Could you check a few things on this model? Use its own coordinates, in mm. A direction names the side the tool comes from. Coordinates: 2 decimals unless noted, no trailing zeros. Loops run counter-clockwise (first coordinate to the right, second up) from the corner with the lowest first, then second, coordinate; pieces in that order, holes last. Notation, with made-up numbers: (-34.75, 34.25) -> (-1.75, 34.25) arc R16 cw to (-1.75, 42.25) -> close; hole circle Ø7 at (76.25, 1.25). An arc over 180 degrees is marked (long way). One line per question, with ' | ' between items.
from build123d import *

# Parameters (mm, degrees)
SKETCH1_W            = 224.79
SKETCH1_H            = 146.05
BOSS_EXTRUDE1_DEPTH  = 1.98374
SKETCH2_W            = 20.32
SKETCH2_H            = 20.32
SKETCH2_H_2          = 1.27
CORNER_CUT_DEPTH     = 135.049326274
SKETCH3_R            = 2.159
PS_MOUNT_HOLES_DEPTH = 135.049326274
PS_CUTOUT_DEPTH      = 135.049326274
FILLET11_R           = 6.35
SKETCH5_R            = 2.8956
FRAME_MOUNTS_DEPTH   = 135.049326274
SKETCH8_W            = 204.47
SKETCH8_H            = 19.05
BOSS_EXTRUDE2_DEPTH  = 1.98374


with BuildPart() as part:
    # Sketch1 → Boss-Extrude1 (new body)
    with BuildSketch(Plane.XY):
        Rectangle(SKETCH1_W, SKETCH1_H)
    extrude(amount=BOSS_EXTRUDE1_DEPTH)

    # Sketch2 → Corner Cut (cut, through all)
    with BuildSketch(Plane.XY.offset(1.98374)):
        with Locations((-102.235, 62.865)):
            Rectangle(SKETCH2_W, SKETCH2_H)
        with Locations((-102.235, -72.39)):
            Rectangle(SKETCH2_W, SKETCH2_H_2)
    extrude(amount=-CORNER_CUT_DEPTH, mode=Mode.SUBTRACT)

    # Sketch3 → PS Mount Holes (cut, through all)
    with BuildSketch(Plane.XY.offset(1.98374)):
        with Locations((-86.075, 46.705)):
            Circle(SKETCH3_R)
        with Locations((-62.0776, -27.295)):
            Circle(SKETCH3_R)
        with Locations((39.925000098, -17.295)):
            Circle(SKETCH3_R)
        with Locations((39.925000098, 46.705)):
            Circle(SKETCH3_R)
    extrude(amount=-PS_MOUNT_HOLES_DEPTH, mode=Mode.SUBTRACT)

    # Sketch4 → PS Cutout (cut, through all)
    with BuildSketch(Plane.XY.offset(1.98374)):
        Polygon((-77.185, 55.595), (31.035000098, 55.595), (31.035000098, 37.815), (48.815000098, 37.815), (48.815000098, -8.405), (31.035000098, -8.405), (31.035000098, -36.185), (-53.1876, -36.185), (-53.1876, -18.405), (-94.965, -18.405), (-94.965, 37.815), (-77.185, 37.815), align=None)
    extrude(amount=-PS_CUTOUT_DEPTH, mode=Mode.SUBTRACT)

    # Fillet11
    fillet11_edges = [part.edges().sort_by_distance(p)[0] for p in [
        (-77.185, 37.815, 0.99187),
        (-77.185, 55.595, 0.99187),
        (31.035000098, 55.595, 0.99187),
        (31.035000098, 37.815, 0.99187),
        (48.815000098, 37.815, 0.99187),
        (48.815000098, -8.405, 0.99187),
        (31.035000098, -8.405, 0.99187),
        (31.035000098, -36.185, 0.99187),
        (-53.1876, -36.185, 0.99187),
        (-53.1876, -18.405, 0.99187),
        (-94.965, -18.405, 0.99187),
        (-94.965, 37.815, 0.99187),
    ]]
    fillet(fillet11_edges, radius=FILLET11_R)

    # Sketch5 → Frame-Mounts (cut, through all)
    with BuildSketch(Plane.XY.offset(1.98374)):
        with Locations((-62.865, 64.77)):
            Circle(SKETCH5_R)
        with Locations((76.835, 64.77)):
            Circle(SKETCH5_R)
        with Locations((-104.14, -36.83)):
            Circle(SKETCH5_R)
    extrude(amount=-FRAME_MOUNTS_DEPTH, mode=Mode.SUBTRACT)

    # Sketch8 → Boss-Extrude2 (add)
    with BuildSketch(Plane.XZ.offset(73.025)):
        with Locations((10.16, -7.54126)):
            Rectangle(SKETCH8_W, SKETCH8_H)
    extrude(amount=BOSS_EXTRUDE2_DEPTH)


solid = part.part
1) On a 3-axis mill with a long thin cutter (end or side, diameter ignored), from which of +Z, -Z, +X, -X, +Y, -Y can I reach the whole of each face in a straight line? I mean faces 1 (the face through (112.395, -1, 1)), 2 (the face through (32.94, 39.63, 0.98)), 3 (the face through (9, -73.025, -8)). Say none if no direction works.
Data:
face 1: +Z, -Z, +X, +Y, -Y | face 2: +Z, -Z | face 3: -Z, +X, -X, +Y
2) If we section it at B-B on y = 64.77: Please give me the cut outline in (x, z) (3 decimals).
Data:
outline: (-92.075, 0) -> (-65.761, 0) -> (-65.761, 1.984) -> (-92.075, 1.984) -> close; (-59.969, 0) -> (73.939, 0) -> (73.939, 1.984) -> (-59.969, 1.984) -> close; (79.731, 0) -> (112.395, 0) -> (112.395, 1.984) -> (79.731, 1.984) -> close
3) If we section it at D-D on x = -26.5: Please give me the cut outline in (y, z) (3 decimals).
Data:
outline: (-75.009, -17.066) -> (-73.025, -17.066) -> (-73.025, 0) -> (-36.185, 0) -> (-36.185, 1.984) -> (-75.009, 1.984) -> close; (55.595, 0) -> (73.025, 0) -> (73.025, 1.984) -> (55.595, 1.984) -> close
4) If we section it at C-C on x = 90.5: Please give me the cut outline in (y, z) (3 decimals).
Data:
outline: (-75.009, -17.066) -> (-73.025, -17.066) -> (-73.025, 0) -> (73.025, 0) -> (73.025, 1.984) -> (-75.009, 1.984) -> close
5) We'd pull the mould along Y, two halves only. Please class faces 4 (the face through (48, -16, 1.984)), 5 (the face through (9, -75.009, -7)), 6 (the face through (47, 35.91, 0.98)): pulls with the +Y half, pulls with the -Y half, needs draft (parallel to the pull), parting line crosses it, or undercut.
Data:
face 4: needs draft | face 5: pulls with the -Y half | face 6: undercut
6) I'm going to push flat-ended pins straight in: pin 1 Ø9.5 at (x, y) = (76.835, 64.77) entering from -Z; pin 2 Ø1.6 at (y, z) = (-74, -7.5) entering from -X (3 decimals); pin 3 Ø5 at (x, z) = (-87, -6.5) entering from +Y (3 decimals). Where does each tip first touch, or does it pass through?
Data:
pin 1: z = 0 | pin 2: x = -92.075 | pin 3: y = -73.025
7) If we section it at A-A on x = -104.14: Please give me the cut outline in (y, z) (3 decimals).
Data:
outline: (-71.755, 0) -> (-39.726, 0) -> (-39.726, 1.984) -> (-71.755, 1.984) -> close; (-33.934, 0) -> (52.705, 0) -> (52.705, 1.984) -> (-33.934, 1.984) -> close
8) I need wall thicknesses on line 1 along Y through (x, z) = (-104.14, 0.55) (3 decimals); line 2 along Y through (x, z) = (-20.5, 1) (3 decimals); line 3 along Y through (x, z) = (72, -14) (3 decimals). Which ranges of each line are inside material? Lowest first, please. Write a range as from..to.
Data:
line 1: -71.755..-39.726, -33.934..52.705 | line 2: -75.009..-36.185, 55.595..73.025 | line 3: -75.009..-73.025
